from build123d import *

# Parameters (mm, degrees)
SKETCH1_W           = 139.7
SKETCH1_H           = 154.20848
BOSS_EXTRUDE1_DEPTH = 6.35
SKETCH2_W           = 127
SKETCH2_H           = 141.50848
CUT_EXTRUDE1_DEPTH  = 6.35
SKETCH3_W           = 139.7
SKETCH3_H           = 154.20848
SKETCH3_W_2         = 134.62
SKETCH3_H_2         = 149.12848
BOSS_EXTRUDE2_DEPTH = 57.15
SKETCH4_W           = 139.7
SKETCH4_H           = 84.35848
CUT_EXTRUDE2_DEPTH  = 64.5
SKETCH5_W           = 2.2225
SKETCH5_H           = 3.175
BOSS_EXTRUDE3_DEPTH = 3.175
FILLET1_R           = 1.5875


with BuildPart() as part:
    # Sketch1 → Boss-Extrude1 (new body)
    with BuildSketch(Plane(origin=(0, 0, 0), x_dir=(1, 0, 0), z_dir=(0, 1, 0))):
        Rectangle(SKETCH1_W, SKETCH1_H)
    extrude(amount=BOSS_EXTRUDE1_DEPTH)

    # Sketch2 → Cut-Extrude1 (cut)
    with BuildSketch(Plane(origin=(0, 6.35, 0), x_dir=(1, 0, 0), z_dir=(0, 1, 0))):
        Rectangle(SKETCH2_W, SKETCH2_H)
    extrude(amount=-CUT_EXTRUDE1_DEPTH, mode=Mode.SUBTRACT)

    # Sketch3 → Boss-Extrude2 (add)
    with BuildSketch(Plane(origin=(0, 6.35, 0), x_dir=(1, 0, 0), z_dir=(0, 1, 0))):
        Rectangle(SKETCH3_W, SKETCH3_H)
        Rectangle(SKETCH3_W_2, SKETCH3_H_2, mode=Mode.SUBTRACT)
    extrude(amount=BOSS_EXTRUDE2_DEPTH)

    # Sketch4 → Cut-Extrude2 (cut, through all)
    with BuildSketch(Plane(origin=(0, 63.5, 0), x_dir=(1, 0, 0), z_dir=(0, 1, 0))):
        with Locations((0, 34.925)):
            Rectangle(SKETCH4_W, SKETCH4_H)
    extrude(amount=-CUT_EXTRUDE2_DEPTH, mode=Mode.SUBTRACT)

    # Sketch5 → Boss-Extrude3 (add)
    with BuildSketch(Plane(origin=(0, 0, 7.25424), x_dir=(-1, 0, 0), z_dir=(0, 0, -1))):
        with Locations((-66.19875, 3.175)):
            Rectangle(SKETCH5_W, SKETCH5_H)
        with Locations((66.19875, 3.175)):
            Rectangle(SKETCH5_W, SKETCH5_H)
    extrude(amount=BOSS_EXTRUDE3_DEPTH)

    # Fillet1
    fillet1_edges = [part.edges().sort_by_distance(p)[0] for p in [
        (-67.31, 34.925, 74.56424),
        (67.31, 34.925, 74.56424),
        (69.85, 31.75, 77.10424),
        (-69.85, 31.75, 77.10424),
    ]]
    fillet(fillet1_edges, radius=FILLET1_R)


solid = part.part
Work out the finished part from the listing and answer in its coordinate system (mm). A direction names the side the tool comes from. Give positions to 0.01 mm unless a question says otherwise; leave off trailing zeros. Loops run counter-clockwise (first coordinate to the right, second up) from the corner with the lowest first, then second, coordinate; pieces in that order, holes last. Notation, with made-up numbers: (55.5, -15) -> (91.5, -15) arc R14 cw to (91.5, 3) -> close; hole circle Ø3 at (58.25, 72.25). An arc over 180 degrees is marked (long way). Use a Markdown table: item, result. Add a question column.
1. Flat-ended cylindrical pins translate along their axes: pin 1 Ø1 at (y, z) = (4, 6) entering from +X; pin 2 Ø6 at (x, y) = (47.5, 8.5) entering from -Z; pin 3 Ø1 at (y, z) = (2.5, 5) entering from -X. Find the tip coordinate at first contact, or state that the pin passes through.
2. Determine the mould class of faces 4 (the flat face through (-1, 3, 70.754)), 5 (the flat face through (-69.85, 31, 42)), 6 (the flat face through (-1, 31, 77.104)) for opening direction X: released by +X, released by -X, zero draft, split by the parting line, or undercut.
3. Section A-A on z = 59.5 is taken. Determine the outline of the cut face in (x, y).
4. Find the intervals of material crossed by probe 1 along X at (y, z) = (34.5, 27); probe 2 along X at (y, z) = (5, 35.5); probe 3 along Z at (x, y) = (43, 28), in increasing order.
5. Section C-C on x = 4.5 is taken. Determine the outline of the cut face in (y, z), and give its area (3 significant figures).
6. For faces 1 (the flat face through (67.31, 35, 41)), 2 (the flat face through (63.5, 3, 39)), 3 (the flat face through (67.31, 3, 6)), determine the directions among +Z, -Z, +X, -X, +Y, -Y from which every point of the face is accessible in a straight line to the end or side of a thin tool.
Results below:
| question | item | result |
|---|---|---|
| 1 | pin 1 | stops at x = 67.31 |
| 1 | pin 2 | stops at z = 70.75 |
| 1 | pin 3 | stops at x = -67.31 |
| 2 | face 4 | undercut |
| 2 | face 5 | released by -X |
| 2 | face 6 | zero draft |
| 3 | outline | (-69.85, 0) -> (-63.5, 0) -> (-63.5, 6.35) -> (-67.31, 6.35) -> (-67.31, 63.5) -> (-69.85, 63.5) -> close; (63.5, 0) -> (69.85, 0) -> (69.85, 63.5) -> (67.31, 63.5) -> (67.31, 6.35) -> (63.5, 6.35) -> close |
| 4 | probe 1 | x = -69.85 to -67.31, 67.31 to 69.85 |
| 4 | probe 2 | x = -69.85 to -63.5, 63.5 to 69.85 |
| 4 | probe 3 | z = 74.56 to 77.1 |
| 5 | outline | (0, 70.75) -> (6.35, 70.75) -> (6.35, 74.56) -> (63.5, 74.56) -> (63.5, 77.1) -> (0, 77.1) -> close |
| 5 | area | 185 mm^2 |
| 6 | face 1 | -Z, +Y |
| 6 | face 2 | -Z, +Y, -Y |
| 6 | face 3 | -Z, +X, +Y, -Y |
